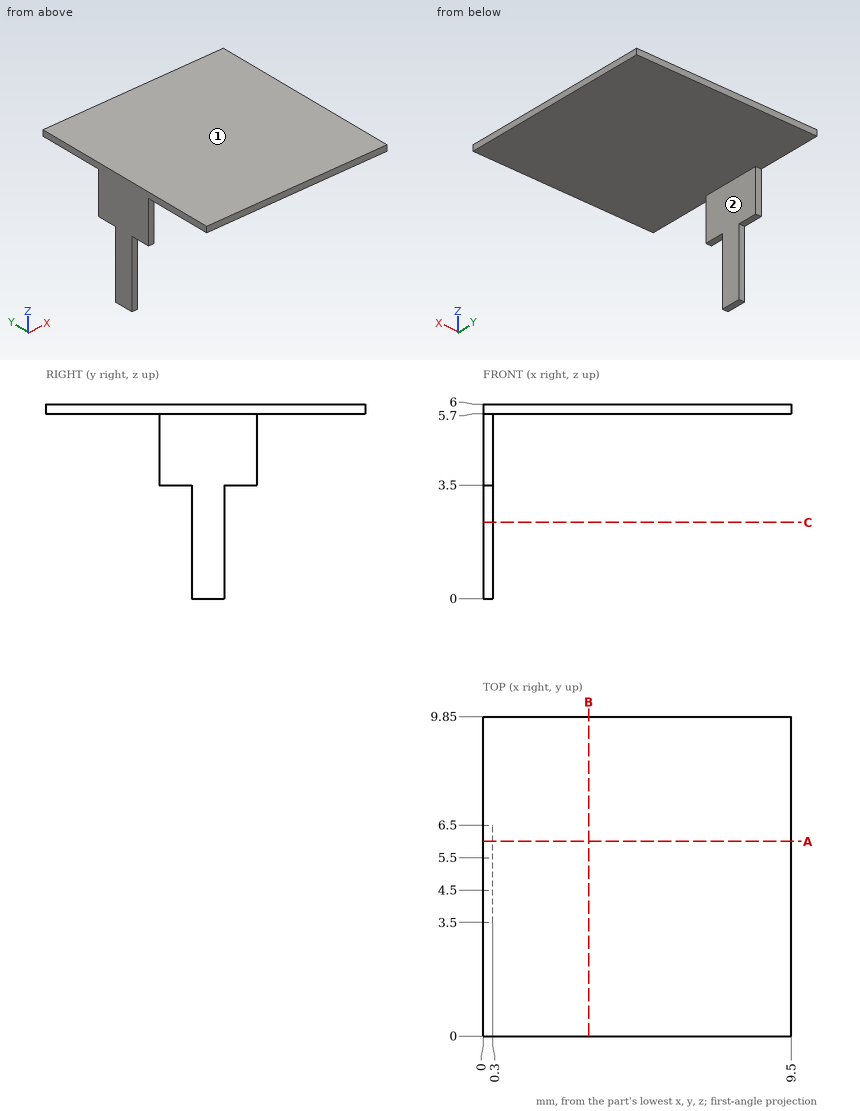
Could you check a few things on this drawing? It's one solid part, dimensions in mm from its lowest x, y, z. A direction names the side the tool comes from. Give positions to 0.01 mm unless a question says otherwise; leave off trailing zeros. Write each loop counter-clockwise with the first axis right and the second up, starting at its lowest first coordinate (ties: lowest second). Pieces come first, ordered by that corner, then holes. Notation, with made-up numbers: (-14.75, 41) -> (-6.75, 41) arc R15 cw to (-6.75, 54) -> close; hole circle Ø7 at (35.5, -30). An arc over 180 degrees is marked (long way). Write item = value, one per line.
(1) I need wall thicknesses on probe 1 along X at (y, z) = (6, 3.95); probe 2 along Z at (x, y) = (5.75, 9.75). Which ranges of each line are inside material? Lowest first, please. Write a range as from..to.
Worked out:
probe_1 = 0..0.3
probe_2 = 5.7..6
(2) For the marked faces 1 and 2, which set-ups out of +Z, -Z, +X, -X, +Y, -Y let a thin tool reach every point of the face, with its end or its side?
Worked out:
face_1 = +Z, +X, -X, +Y, -Y
face_2 = -Z, +X, +Y, -Y
(3) Suppose I cut it at A-A on y = 6. Write out the boundary of the cut face in (x, z), then the cut area to 3 significant figures.
Worked out:
outline = (0, 3.5) -> (0.3, 3.5) -> (0.3, 5.7) -> (9.5, 5.7) -> (9.5, 6) -> (0, 6) -> close
area = 3.51 mm^2
(4) I'm going to push a flat-ended pin straight in: P1, Ø1, axis at y = 5.5, z = 1, coming from the +X side. Where does the tip first touch, or does it pass through?
Worked out:
P1 = 0.3
(5) Suppose I cut it at C-C on z = 2.35. Write out the boundary of the cut face in (x, y).
Worked out:
outline = (0, 4.5) -> (0.3, 4.5) -> (0.3, 5.5) -> (0, 5.5) -> close
(6) Suppose I cut it at B-B on x = 3.25. Write out the boundary of the cut face in (y, z).
Worked out:
outline = (0, 5.7) -> (9.85, 5.7) -> (9.85, 6) -> (0, 6) -> close
